from build123d import *

# Parameters (mm, degrees)
SKETCH_2_W      = 69
SKETCH_2_H      = 37
SKETCH_2_R      = 3
EXTRUDE_1_DEPTH = 2
SKETCH_3_W      = 2
SKETCH_3_H      = 37
SKETCH_3_R      = 1.5
SKETCH_3_R_2    = 6
EXTRUDE_2_DEPTH = 4


with BuildPart() as part:
    # 草图2 → 凸台-拉伸1 (new body)
    with BuildSketch(Plane.XY):
        Rectangle(SKETCH_2_W, SKETCH_2_H)
        with Locations((25.25, 9.25)):
            Circle(SKETCH_2_R, mode=Mode.SUBTRACT)
        with Locations(Location((25.25, -9.25, 0), (0, 0, 180))):
            Circle(SKETCH_2_R, mode=Mode.SUBTRACT)
        with Locations(Location((-25.25, 9.25, 0), (0, 0, 180))):
            Circle(SKETCH_2_R, mode=Mode.SUBTRACT)
        with Locations((-25.25, -9.25)):
            Circle(SKETCH_2_R, mode=Mode.SUBTRACT)
    extrude(amount=EXTRUDE_1_DEPTH)

    # 草图3 → 凸台-拉伸2 (add)
    # profile 1 of 3: a face of its own
    with BuildSketch(Plane(origin=(34.5, 0, 0), x_dir=(0, 0, -1), z_dir=(1, 0, 0))):
        with BuildLine():
            ThreePointArc((22.5, -18.5), (4, 0), (22.5, 18.5))
            Line((22.5, 18.5), (0, 18.5))
            Line((0, 18.5), (0, -18.5))
            Line((0, -18.5), (22.5, -18.5))
        make_face()
    # profile 2 of 3: a face of its own
    with BuildSketch(Plane(origin=(34.5, 0, 0), x_dir=(0, 0, -1), z_dir=(1, 0, 0))):
        with Locations((-1, 0)):
            Rectangle(SKETCH_3_W, SKETCH_3_H)
    # profile 3 of 3: a face of its own
    with BuildSketch(Plane(origin=(34.5, 0, 0), x_dir=(0, 0, -1), z_dir=(1, 0, 0))):
        with BuildLine():
            ThreePointArc((41, 0), (35.581475452, 13.081475452), (22.5, 18.5))
            ThreePointArc((22.5, 18.5), (4, 0), (22.5, -18.5))
            ThreePointArc((22.5, -18.5), (35.581475452, -13.081475452), (41, 0))
        make_face()
        with Locations(Location((9.076606241, -7.75, 0), (0, 0, 90))):
            Circle(SKETCH_3_R, mode=Mode.SUBTRACT)
        with Locations(Location((22.5, -15.5, 0), (0, 0, 90))):
            Circle(SKETCH_3_R, mode=Mode.SUBTRACT)
        with Locations(Location((35.923393759, -7.75, 0), (0, 0, 90))):
            Circle(SKETCH_3_R, mode=Mode.SUBTRACT)
        with Locations(Location((15.5, 0, 0), (0, 0, 90))):
            Circle(SKETCH_3_R_2, mode=Mode.SUBTRACT)
        with Locations(Location((9.076606241, 7.75, 0), (0, 0, 90))):
            Circle(SKETCH_3_R, mode=Mode.SUBTRACT)
        with Locations(Location((35.923393759, 7.75, 0), (0, 0, 90))):
            Circle(SKETCH_3_R, mode=Mode.SUBTRACT)
        with Locations(Location((22.5, 15.5, 0), (0, 0, 90))):
            Circle(SKETCH_3_R, mode=Mode.SUBTRACT)
    extrude(amount=EXTRUDE_2_DEPTH)


solid = part.part
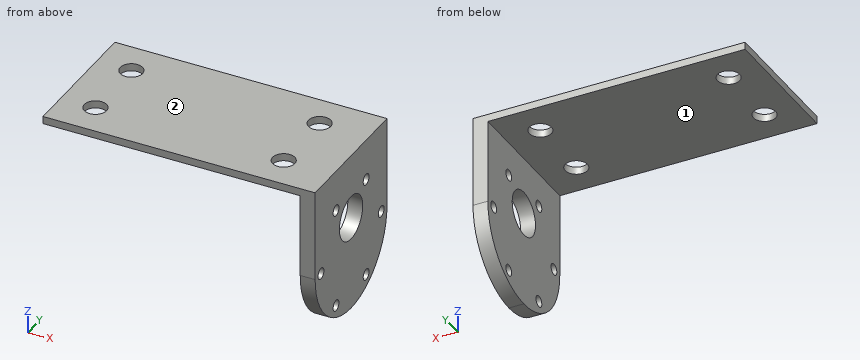
The model under review builds one solid part; all positions refer to its coordinate system, in mm. Face numbers are marked on the shaded views. A direction names the side the tool comes from. Round coordinates to 2 decimals unless told otherwise and drop trailing zeros. Loops run counter-clockwise (first coordinate to the right, second up) from the corner with the lowest first, then second, coordinate; pieces in that order, holes last. Notation, with made-up numbers: (74.5, -1) -> (101.5, -1) arc R30 cw to (101.5, 29) -> close; hole circle Ø8 at (50.5, 57). An arc over 180 degrees is marked (long way). Return JSON: item names as keys, results as strings.
(1) For the marked faces 1 and 2, list the 3-axis set-ups (+Z, -Z, +X, -X, +Y, -Y) from which the entire face can be reached by the end or side of a thin tool; tool diameter is ignored.
Solved:
{"face 1": "-Z, -X, +Y, -Y", "face 2": "+Z, +X, -X, +Y, -Y"}
(2) Add section A-A on z = -15.5. Write out the cut boundary in (x, y), plus the area to 3 significant figures.
Solved:
{"outline": "(34.5, -18.5) -> (38.5, -18.5) -> (38.5, -6) -> (34.5, -6) -> close; (34.5, 6) -> (38.5, 6) -> (38.5, 18.5) -> (34.5, 18.5) -> close", "area": "100 mm2"}
(3) Add section C-C on y = 15.5. Write out the cut boundary in (x, z), plus the area to 3 significant figures.
Solved:
{"outline": "(-34.5, 0) -> (34.5, 0) -> (34.5, -21) -> (38.5, -21) -> (38.5, 2) -> (-34.5, 2) -> close; (34.5, -32.6) -> (38.5, -32.6) -> (38.5, -24) -> (34.5, -24) -> close", "area": "264 mm2"}
(4) For pin 1 (5.5 mm diameter, centred on x = 25.25, y = -9.25, fed in from -Z); pin 2 (18.5 mm diameter, centred on x = 7.5, y = -8, fed in from -Z); pin 3 (5 mm diameter, centred on y = -15.5, z = -22.5, fed in from -X); pin 4 (9.5 mm diameter, centred on x = -25.25, y = -9.25, fed in from +Z), all flat-tipped, find the tip position at first contact; note any pin that passes through.
Solved:
{"pin 1": "through", "pin 2": "z = 0", "pin 3": "x = 34.5", "pin 4": "z = 2"}
(5) Add section D-D on y = -11. Write out the cut boundary in (x, z).
Solved:
{"outline": "(-34.5, 0) -> (-27.69, 0) -> (-27.69, 2) -> (-34.5, 2) -> close; (-22.81, 0) -> (22.81, 0) -> (22.81, 2) -> (-22.81, 2) -> close; (27.69, 0) -> (34.5, 0) -> (34.5, -37.37) -> (38.5, -37.37) -> (38.5, 2) -> (27.69, 2) -> close"}
(6) Add section B-B on x = 25.25. Write out the cut boundary in (y, z), plus the area to 3 significant figures.
Solved:
{"outline": "(-18.5, 0) -> (-12.25, 0) -> (-12.25, 2) -> (-18.5, 2) -> close; (-6.25, 0) -> (6.25, 0) -> (6.25, 2) -> (-6.25, 2) -> close; (12.25, 0) -> (18.5, 0) -> (18.5, 2) -> (12.25, 2) -> close", "area": "50.0 mm2"}
(7) For line 1 (Z direction, x = 36.5, y = 0); line 2 (X direction, y = -6, z = -1.5); line 3 (Z direction, x = -22, y = 12), list the stretches that pass through material, from the lowest coordinate up.
Solved:
{"line 1": "-41 to -21.5, -9.5 to 2", "line 2": "34.5 to 38.5", "line 3": "0 to 2"}
